Verification items for the finished model (mm, model axes). A direction names the side the tool comes from. Give positions to 0.01 mm unless a question says otherwise; leave off trailing zeros. Write each loop counter-clockwise with the first axis right and the second up, starting at its lowest first coordinate (ties: lowest second). Pieces come first, ordered by that corner, then holes. Notation, with made-up numbers: (77, -21) - (88, -21) arc R18 cw to (88, 9) - close; hole circle Ø1 at (13.5, 42). An arc over 180 degrees is marked (long way). Answer as a JSON object with one key per item and string values. Group by question number.
Item 1: Draft check along X on faces 4 (the face through (-12.7, 95, 3)), 5 (the face through (-6, 63.5, 3)), 6 (the face through (27.418, 14.298, 3.219)). Enter one of: +X half, -X half, draft (parallel to the pull), parting line (faces both ways), or undercut.
Item 2: Scan lines: line 1 along Y through (x, z) = (23, 1.5); line 2 along X through (y, z) = (50, 5.5); line 3 along X through (y, z) = (10.5, 4.25). Record each from-to range of solid material in increasing order. Write a range as [from, to].
Item 3: Sectioned sample at C-C, the plane y = 95.25. Record the boundary of the cut face in (x, z), and give its area (3 significant figures).
Item 4: Tool access check on faces 1 (the face through (69.85, 32, 3)), 2 (the face through (16, 9.995, 3)), 3 (the face through (0, 31, 3)). Record the directions out of +Z, -Z, +X, -X, +Y, -Y that give a thin tool (end or side, any length) a straight path to the whole face; none if there is none.
Item 5: Go/stop test with flat-tipped pins: pin 1 (10 mm diameter, centred on x = 67, y = 25.5, fed in from -Z); pin 2 (3 mm diameter, centred on x = -6.5, z = 4, fed in from -Y); pin 3 (3 mm diameter, centred on y = 43.5, z = 5, fed in from -X); pin 4 (5.5 mm diameter, centred on x = -4.572, y = 95.25, fed in from -Z). Record where each tip stops, or that it passes through.
Item 6: Sectioned sample at B-B, the plane x = 18. Record the boundary of the cut face in (y, z), and give its area (3 significant figures).
Item 7: Sectioned sample at D-D, the plane x = 73. Record the boundary of the cut face in (y, z), and give its area (3 significant figures).
Item 8: Sectioned sample at A-A, the plane z = 4.5. Count the separate pieces of the cut face and the enclosed holes in it, and give its area (3 significant figures).
```python
from build123d import *

# Parameters (mm, degrees)
BOSS_EXTRUDE1_DEPTH = 6.35
CUT_EXTRUDE1_REACH  = 153.604
SKETCH2_R           = 3.175
CUT_EXTRUDE2_REACH  = 153.604
FILLET1_R           = 5


with BuildPart() as part:
    # Sketch1 → Boss-Extrude1 (new body)
    with BuildSketch(Plane.XY):
        Polygon((0, 0), (0, 63.5), (-12.7, 63.5), (-12.7, 127), (82.55, 127), (82.55, 63.5), (69.85, 63.5), (69.85, 0), align=None)
    extrude(amount=BOSS_EXTRUDE1_DEPTH)

    # Sketch2 → Cut-Extrude1 (cut, up to next)
    with BuildSketch(Plane.XY.offset(6.35), mode=Mode.PRIVATE) as cut_extrude1_sk1:
        with Locations((-4.572, 95.25)):
            Circle(SKETCH2_R)
    cut_extrude1_tool1 = extrude(cut_extrude1_sk1.sketch, amount=-CUT_EXTRUDE1_REACH, mode=Mode.PRIVATE) & part.part
    # Sketch2 → Cut-Extrude1 (cut, up to next)
    with BuildSketch(Plane.XY.offset(6.35), mode=Mode.PRIVATE) as cut_extrude1_sk2:
        with Locations(Location((74.422, 95.25, 0), (0, 0, 180))):
            Circle(SKETCH2_R)
    cut_extrude1_tool2 = extrude(cut_extrude1_sk2.sketch, amount=-CUT_EXTRUDE1_REACH, mode=Mode.PRIVATE) & part.part
    add(cut_extrude1_tool1.solids().sort_by_distance((-4.572, 95.25, 6.35))[0], mode=Mode.SUBTRACT)
    add(cut_extrude1_tool2.solids().sort_by_distance((74.422, 95.25, 6.35))[0], mode=Mode.SUBTRACT)

    # Sketch3 → Cut-Extrude2 (cut, up to next)
    with BuildSketch(Plane.XY.offset(6.35), mode=Mode.PRIVATE) as cut_extrude2_sk1:
        with BuildLine():
            Line((9.925, 53.50542107), (23.01875, 53.50542107))
            ThreePointArc((23.01875, 53.50542107), (27.41875, 49.10542107), (23.01875, 44.70542107))
            Line((23.01875, 44.70542107), (9.925, 44.70542107))
            ThreePointArc((9.925, 44.70542107), (5.525, 49.10542107), (9.925, 53.50542107))
        make_face()
    cut_extrude2_tool1 = extrude(cut_extrude2_sk1.sketch, amount=-CUT_EXTRUDE2_REACH, mode=Mode.PRIVATE) & part.part
    # Sketch3 → Cut-Extrude2 (cut, up to next)
    with BuildSketch(Plane.XY.offset(6.35), mode=Mode.PRIVATE) as cut_extrude2_sk2:
        with BuildLine():
            Line((59.925, 53.50542107), (46.83125, 53.50542107))
            ThreePointArc((46.83125, 53.50542107), (42.43125, 49.10542107), (46.83125, 44.70542107))
            Line((46.83125, 44.70542107), (59.925, 44.70542107))
            ThreePointArc((59.925, 44.70542107), (64.325, 49.10542107), (59.925, 53.50542107))
        make_face()
    cut_extrude2_tool2 = extrude(cut_extrude2_sk2.sketch, amount=-CUT_EXTRUDE2_REACH, mode=Mode.PRIVATE) & part.part
    # Sketch3 → Cut-Extrude2 (cut, up to next)
    with BuildSketch(Plane.XY.offset(6.35), mode=Mode.PRIVATE) as cut_extrude2_sk3:
        with BuildLine():
            Line((59.925, 9.99457893), (46.83125, 9.99457893))
            ThreePointArc((46.83125, 9.99457893), (42.43125, 14.39457893), (46.83125, 18.79457893))
            Line((46.83125, 18.79457893), (59.925, 18.79457893))
            ThreePointArc((59.925, 18.79457893), (64.325, 14.39457893), (59.925, 9.99457893))
        make_face()
    cut_extrude2_tool3 = extrude(cut_extrude2_sk3.sketch, amount=-CUT_EXTRUDE2_REACH, mode=Mode.PRIVATE) & part.part
    # Sketch3 → Cut-Extrude2 (cut, up to next)
    with BuildSketch(Plane.XY.offset(6.35), mode=Mode.PRIVATE) as cut_extrude2_sk4:
        with BuildLine():
            Line((9.925, 9.99457893), (23.01875, 9.99457893))
            ThreePointArc((23.01875, 9.99457893), (27.41875, 14.39457893), (23.01875, 18.79457893))
            Line((23.01875, 18.79457893), (9.925, 18.79457893))
            ThreePointArc((9.925, 18.79457893), (5.525, 14.39457893), (9.925, 9.99457893))
        make_face()
    cut_extrude2_tool4 = extrude(cut_extrude2_sk4.sketch, amount=-CUT_EXTRUDE2_REACH, mode=Mode.PRIVATE) & part.part
    add(cut_extrude2_tool1.solids().sort_by_distance((16.471875, 49.105421, 6.35))[0], mode=Mode.SUBTRACT)
    add(cut_extrude2_tool2.solids().sort_by_distance((53.378125, 49.105421, 6.35))[0], mode=Mode.SUBTRACT)
    add(cut_extrude2_tool3.solids().sort_by_distance((53.378125, 14.394579, 6.35))[0], mode=Mode.SUBTRACT)
    add(cut_extrude2_tool4.solids().sort_by_distance((16.471875, 14.394579, 6.35))[0], mode=Mode.SUBTRACT)

    # Fillet1
    fillet1_edges = [part.edges().sort_by_distance(p)[0] for p in [
        (0, 0, 3.175),
        (0, 63.5, 3.175),
        (-12.7, 63.5, 3.175),
        (-12.7, 127, 3.175),
        (82.55, 127, 3.175),
        (82.55, 63.5, 3.175),
        (69.85, 63.5, 3.175),
        (69.85, 0, 3.175),
    ]]
    fillet(fillet1_edges, radius=FILLET1_R)


solid = part.part
```
Geometry check:
{
 "1": {"face 4": "-X half", "face 5": "draft", "face 6": "undercut"},
 "2": {"line 1": "[0, 9.99], [18.79, 44.71], [53.51, 127]", "line 2": "[0, 5.62], [27.33, 42.52], [64.23, 69.85]", "line 3": "[0, 7.88], [25.07, 44.78], [61.97, 69.85]"},
 "3": {"outline": "(-12.7, 0) - (-7.75, 0) - (-7.75, 6.35) - (-12.7, 6.35) - close; (-1.4, 0) - (71.25, 0) - (71.25, 6.35) - (-1.4, 6.35) - close; (77.6, 0) - (82.55, 0) - (82.55, 6.35) - (77.6, 6.35) - close", "area": "524 mm^2"},
 "4": {"face 1": "+Z, -Z, +X, -Y", "face 2": "+Z, -Z", "face 3": "+Z, -Z, -X, -Y"},
 "5": {"pin 1": "z = 0", "pin 2": "y = 63.5", "pin 3": "x = 0", "pin 4": "through"},
 "6": {"outline": "(0, 0) - (9.99, 0) - (9.99, 6.35) - (0, 6.35) - close; (18.79, 0) - (44.71, 0) - (44.71, 6.35) - (18.79, 6.35) - close; (53.51, 0) - (127, 0) - (127, 6.35) - (53.51, 6.35) - close", "area": "695 mm^2"},
 "7": {"outline": "(63.15, 0) - (92.41, 0) - (92.41, 6.35) - (63.15, 6.35) - close; (98.09, 0) - (127, 0) - (127, 6.35) - (98.09, 6.35) - close", "area": "369 mm^2"},
 "8": {"separate pieces": "1", "enclosed holes": "6", "area": "9,690 mm^2"}
}
